Autodesk Inventor part; units mm, degrees
ref_plane "YZ Plane" through (0, 0, 0) normal (1, 0, 0) x (0, 1, 0)
ref_plane "XZ Plane" through (0, 0, 0) normal (0, 1, 0) x (-1, 0, 0)
ref_plane "XY Plane" through (0, 0, 0) normal (0, 0, 1) x (1, 0, 0)
ref_plane "Plano de trabajo1" through (0, 0, 0) normal (0, 0, 1) x (1, 0, 0)
sketch "Boceto1" plane through (0, 0, 0) normal (0, 0, 1) x (1, 0, 0)
  circle A0 centre (-9.9048, 81.1277) radius 6.5
  line L0 (-79.9048, 100.693) -> (-79.9048, 87.6277)
  line L1 (-79.9048, 74.6277) -> (-79.9048, 61.5627)
  line L2 (-79.9048, 87.6277) -> (-79.9048, 74.6277)
  circle A1 centre (-9.9048, 81.1277) radius 9
  line L3 (-79.9048, 100.693) -> (-9.9048, 90.1277)
  line L4 (-79.9048, 61.5627) -> (-9.9048, 72.1277)
  point P0 (0, 0)
  dimension "d0" = 13
  dimension "d2" = 13.065
  dimension "d3" = 18
extrude "Extrusión1" add sketch "Boceto1" along normal blind 20
sketch "Boceto2" plane through (-79.9048, 61.5627, 0) normal (-1, 0, 0) x (0, 0, 1)
  line L0 (0, 39.1303) -> (0, 0)
  line L1 (20, 39.1303) -> (20, 0)
  line L2 (0, 39.1303) -> (20, 0)
  line L3 (20, 39.1303) -> (0, 0)
  line L4 (40, -0.4348) -> (-20, -0.4348)
  line L5 (-20, -0.4348) -> (-20, 39.5652)
  line L6 (-20, 39.5652) -> (40, 39.5652)
  line L7 (40, 39.5652) -> (40, -0.4348)
  line L8 (40, -0.4348) -> (-20, 39.5652) construction
  line L9 (-20, -0.4348) -> (40, 39.5652) construction
  point P0 (0, -61.5627)
  point P1 (10, 19.5652)
  dimension "d6" = 60
  dimension "d7" = 40
extrude "Extrusión2" add sketch "Boceto2" along normal blind 3 contours L2 L3 L0 | L3 L1 L2 | L4 L5 L6 L7
fillet "Empalme1" radius 2 4 edges at (-81.4048, 101.1278, -20) (-81.4048, 101.1278, 40) (-81.4048, 61.1278, -20) (-81.4048, 61.1278, 40)
sketch "Boceto4" plane through (-82.9048, 61.5627, 0) normal (-1, 0, 0) x (0, 0, 1)
  line L0 (-10.1021, 39.6035) -> (-10.1021, 29.6035)
  line L1 (-10.1021, 29.6035) -> (-20.1021, 29.6035)
  circle A0 centre (-10.1021, 29.6035) radius 1.7
  line L2 (-10.1021, 29.6035) -> (-10.1021, -0.4348)
  line L3 (38, -0.4348) -> (-18, -0.4348)
  line L4 (-10.1021, -0.4348) -> (-10.1021, 9.5652)
  line L5 (-10.1021, 9.5652) -> (40.1083, 9.5652)
  line L6 (40.1083, 9.5652) -> (30.1083, 9.5652)
  line L7 (30.1083, 9.5652) -> (30.1083, 39.6035)
  line L8 (30.1083, 39.6035) -> (30.1083, 29.6035)
  circle A1 centre (-10.1021, 9.5652) radius 1.7
  circle A2 centre (30.1083, 9.5652) radius 1.7
  circle A3 centre (30.1083, 29.6035) radius 1.7
  point P0 (0, -61.5627)
  dimension "d11" = 10
  dimension "d12" = 10
  dimension "d13" = 3.4
  dimension "d14" = 10
  dimension "d15" = 10
  dimension "d16" = 10
  dimension "d17" = 3.4
  dimension "d18" = 3.4
  dimension "d19" = 3.4
extrude "Extrusión3" cut sketch "Boceto4" against normal blind 3
sketch "Boceto5" plane through (0, 0, 20) normal (0, 0, 1) x (1, 0, 0)
  circle A0 centre (-9.8912, 81.0888) radius 7
  point P0 (0, 0)
  dimension "d22" = 14
extrude "Extrusión4" add sketch "Boceto5" against normal blind 5
sketch "Boceto6" plane through (0, 0, 0) normal (0, 0, -1) x (-1, 0, 0)
  circle A0 centre (-4.1803, 81.1277) radius 12.4106
  point P0 (0, 0)
extrude "Extrusión5" cut sketch "Boceto6" against normal blind 20
fillet "Empalme2" radius 0.5 5 edges at (-6.83, 75.4009, 7.5) (-6.83, 86.8544, 7.5) (-5.4544, 88.9504, 10) (-5.4544, 73.305, 10) (-8.2303, 81.1277, 20)
properties part number "soporte"
For this review, take the finished solid that the model builds, in its own axes (mm). A direction names the side the tool comes from. Round coordinates to 2 decimals unless told otherwise and drop trailing zeros. Loops run counter-clockwise (first coordinate to the right, second up) from the corner with the lowest first, then second, coordinate; pieces in that order, holes last. Notation, with made-up numbers: (62.5, 18) - (83.5, 18) arc R23 cw to (83.5, 45) - close; hole circle Ø9 at (81, 75.5). An arc over 180 degrees is marked (long way). Put each result on its own line as item: value. Start each with the question number.
1. Mouldability with a two-part tool opening along Y and no side actions: class faces 1 (the flat face through (-45.395, 95.484, 9.86)), 2 (the cylindrical face through (-8.23, 81.02, 16.11)), 3 (the flat face through (-45.39, 66.77, 9.86)), 4 (the cylindrical face through (-81.43, 72.28, 28.86)) as +Y half, -Y half, draft (parallel to the pull), parting line (faces both ways), or undercut.
2. Insertion check: P1, Ø3, axis at x = -37, y = 79.5, coming from the +Z side; P2, Ø5.5, axis at y = 71.13, z = -10.1, coming from the +X side; P3, Ø10, axis at x = -28, y = 85, coming from the -Z side. Each pin has a flat end and moves straight along its axis. Give the tip position at first contact, or say it passes through.
3. Consider section B-B on z = -3.5. State the section outline as (x, y) points.
4. Consider section A-A on y = 66. State the section outline as (x, z) points.
5. For probe 1 along Z at (x, y) = (-34, 81); probe 2 along X at (y, z) = (78.5, 21.5); probe 3 along X at (y, z) = (73.5, 17), list the stretches that pass through material, from the lowest coordinate up. Write a range as [from, to].
6. Consider section C-C on x = -70. State the section outline as (y, z) points.
7. For faces 5 (the cylindrical face through (-81.426, 72.813, -10.323)), 6 (the flat face through (-52, 81, 0)), 7 (the flat face through (-52, 81, 20)), list the 3-axis set-ups (+Z, -Z, +X, -X, +Y, -Y) from which the entire face can be reached by the end or side of a thin tool; tool diameter is ignored.
Result sheet:
1. face 1: +Y half
1. face 2: undercut
1. face 3: -Y half
1. face 4: undercut
2. P1: z = 20
2. P2: x = -79.9
2. P3: z = 0
3. outline: (-82.9, 61.13) - (-79.9, 61.13) - (-79.9, 101.13) - (-82.9, 101.13) - close
4. outline: (-82.9, -20) - (-79.9, -20) - (-79.9, 0) - (-50.5, 0) - (-50.5, 20) - (-79.9, 20) - (-79.9, 40) - (-82.9, 40) - close
5. probe 1: [0, 20]
5. probe 2: [-82.9, -79.9]
5. probe 3: [-82.9, -5.72]
6. outline: (63.06, 0) - (99.2, 0) - (99.2, 20) - (63.06, 20) - close
7. face 5: +X, -X
7. face 6: -Z, +X, +Y, -Y
7. face 7: +Z, +X, +Y, -Y
